from build123d import *

# Parameters (mm, degrees)
SKETCH1_R           = 5
BOSS_EXTRUDE1_DEPTH = 7
SKETCH2_R           = 3.5
CUT_EXTRUDE1_DEPTH  = 10.949874371
BOSS_EXTRUDE4_START = 1.6
SKETCH3_R           = 4
SKETCH3_R_2         = 3.5
BOSS_EXTRUDE4_DEPTH = 1.6


with BuildPart() as part:
    # Sketch1 → Boss-Extrude1 (new body)
    with BuildSketch(Plane.XY):
        Circle(SKETCH1_R)
    extrude(amount=BOSS_EXTRUDE1_DEPTH)

    # Sketch2 → Cut-Extrude1 (cut, through all)
    with BuildSketch(Plane.XY.offset(7)):
        Circle(SKETCH2_R)
    extrude(amount=-CUT_EXTRUDE1_DEPTH, mode=Mode.SUBTRACT)

    # Sketch3 → Boss-Extrude4 (add)
    with BuildSketch(Plane.XY.offset(7).offset(BOSS_EXTRUDE4_START)):
        Circle(SKETCH3_R)
        Circle(SKETCH3_R_2, mode=Mode.SUBTRACT)
    extrude(amount=-BOSS_EXTRUDE4_DEPTH)


solid = part.part
Source: CAD feature listing. Evaluate the final solid. Frame: model axes, mm. Round coordinates to 2 decimals unless told otherwise and drop trailing zeros. Write each loop counter-clockwise with the first axis right and the second up, starting at its lowest first coordinate (ties: lowest second). Pieces come first, ordered by that corner, then holes. Notation, with made-up numbers: M 17.5,89.5 L 53.5,89.5 A29 ccw 53.5,127.5 Z; hole C -32.5,26 d3. An arc over 180 degrees is marked long. One line per item, written item: value. Start each with the question number.
Item 1: Section query D-D (y = 4.25). Return the cut outline in (x, z).
Item 2: Section query A-A (x = 0). Return the cut outline in (y, z).
Item 3: Mould query, pull axis Y, two halves, no side actions, for faces 1 (the cylindrical face through (3.233, -1.341, 4.36)), 2 (the flat face through (2.2, -3.3, 0)), 3 (the cylindrical face through (-1.08, -4.88, 3.45)). Classes: pulls with the +Y half, pulls with the -Y half, needs draft (parallel to the pull), parting line crosses it, or undercut.
Item 4: Section query C-C (z = 6). Return the cut outline in (x, y), plus the area to 3 significant figures.
Item 5: Ray query, L1, parallel to Y at x = 0, z = 2.5; L2, parallel to Z at x = -3, y = 3.75; L3, parallel to X at y = -0.5, z = 4.25. Return the intervals inside material, ascending. Write a range as from..to.
Item 6: Pin query (flat end, axial travel): pin 1 (1.5 mm diameter, centred on x = 4, z = 7, fed in from +Y); pin 2 (4 mm diameter, centred on x = 2.5, z = 6, fed in from -Y). Return the tip coordinate at first contact, or that it passes through.
Result set:
1. outline: M -2.63,0 L 2.63,0 L 2.63,7 L -2.63,7 Z
2. outline: M -5,0 L -3.5,0 L -3.5,8.6 L -4,8.6 L -4,7 L -5,7 Z; M 3.5,0 L 5,0 L 5,7 L 4,7 L 4,8.6 L 3.5,8.6 Z
3. face 1: undercut
3. face 2: needs draft
3. face 3: parting line crosses it
4. outline: C 0,0 d10; hole C 0,0 d7
4. area: 40.1 mm²
5. L1: y = -5..-3.5, 3.5..5
5. L2: z = 0..7
5. L3: x = -4.97..-3.46, 3.46..4.97
6. pin 1: stops at y = 3.8
6. pin 2: stops at y = -4.97
